Part print with two shaded views. Sizes in mm from the minimum x, y, z corner. A direction names the side the tool comes from. Give positions to 0.01 mm unless a question says otherwise; leave off trailing zeros. Write each loop counter-clockwise with the first axis right and the second up, starting at its lowest first coordinate (ties: lowest second). Pieces come first, ordered by that corner, then holes. Notation, with made-up numbers: (15, -35.75) -> (22, -35.75) arc R22 ccw to (22, 2.25) -> close; hole circle Ø7 at (-34.5, 36). An arc over 180 degrees is marked (long way). Write item = value, one per line. Start each with the question number.
Q1. Saw through at B-B, the plane z = 6. List the corners of the cut face in (x, y).
Q2. Wall check: line 1 (Y direction, x = 56, z = 45); line 2 (X direction, y = 13, z = 3); line 3 (Z direction, x = 18, y = 26.5). Give the ranges that are in metal, low to high.
Q3. Tool access for the marked faces 1, 2 and 3: list every direction of +Z, -Z, +X, -X, +Y, -Y with a clear straight run to the whole face (end or side of a thin tool).
Q4. Drop flat-ended pins along their axis: P1, Ø1.5, axis at x = 14, y = 29.5, coming from the -Z side; P2, Ø17.5, axis at x = 60, z = 12, coming from the -Y side; P3, Ø14, axis at x = 55, z = 42, coming from the -Y side; P4, Ø10, axis at x = 37, y = 34, coming from the +Z side. Give the stop position or say it passes through.
Q5. Saw through at A-A, the plane y = 53. List the corners of the cut face in (x, z).
Q6. Saw through at C-C, the plane x = 7.5. List the corners of the cut face in (y, z), then the cut area to 3 significant figures.
Q7. Saw through at D-D, the plane y = 16. List the corners of the cut face in (x, z).
Q8. Mould opens along X. For the marked faces 4, 5, 6 and 7 say: pulls with the +X half, pulls with the -X half, needs draft (parallel to the pull), parting line crosses it, or undercut.
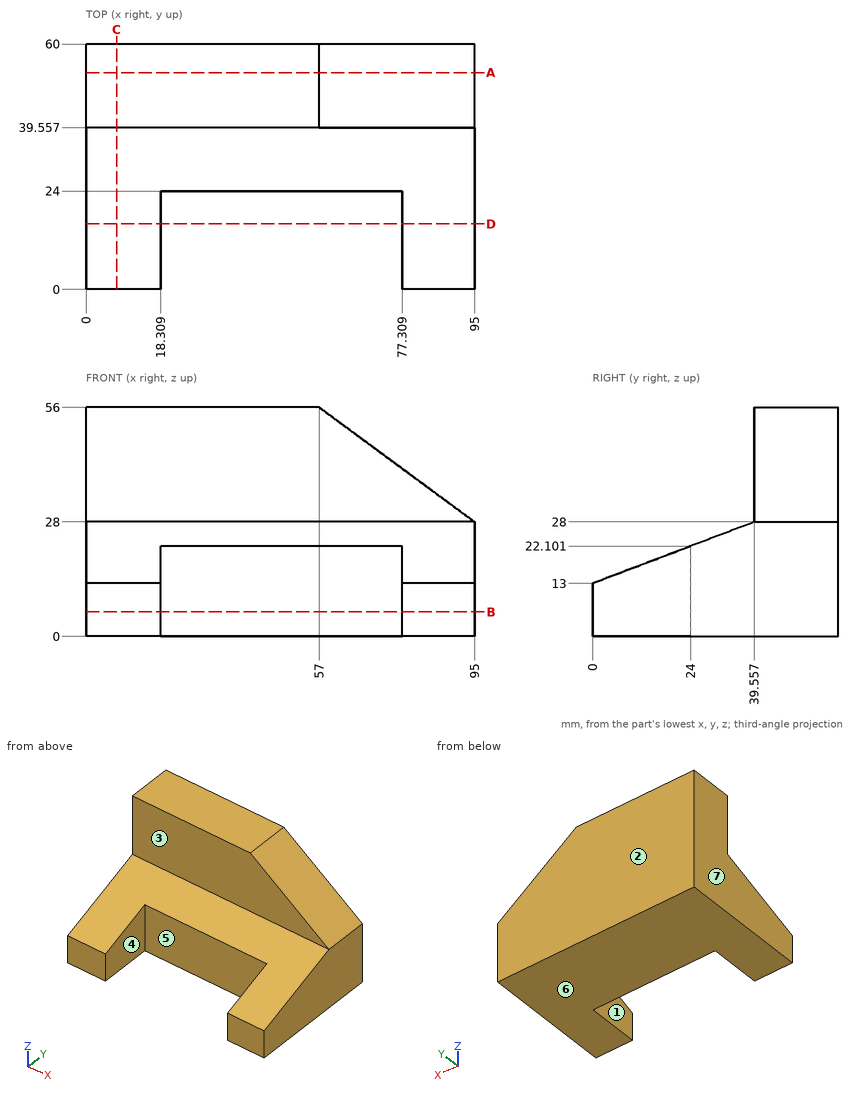
Report:
q1.outline = (0, 0) -> (18.31, 0) -> (18.31, 24) -> (77.31, 24) -> (77.31, 0) -> (95, 0) -> (95, 60) -> (0, 60) -> close
q2.line_1 = 39.56 to 60
q2.line_2 = 0 to 18.31, 77.31 to 95
q2.line_3 = 0 to 23.05
q3.face_1 = +Z, -Z, -Y
q3.face_2 = +Z, -Z, +X, -X, +Y
q3.face_3 = +Z, +X, -X, -Y
q4.P1 = 0
q4.P2 = 24
q4.P3 = 39.56
q4.P4 = 27.79
q5.outline = (0, 0) -> (95, 0) -> (95, 28) -> (57, 56) -> (0, 56) -> close
q6.outline = (0, 0) -> (60, 0) -> (60, 56) -> (39.56, 56) -> (39.56, 28) -> (0, 13) -> close
q6.area = 1,960 mm2
q7.outline = (0, 0) -> (18.31, 0) -> (18.31, 19.07) -> (0, 19.07) -> close; (77.31, 0) -> (95, 0) -> (95, 19.07) -> (77.31, 19.07) -> close
q8.face_4 = undercut
q8.face_5 = undercut
q8.face_6 = needs draft
q8.face_7 = pulls with the -X half
